```python
from build123d import *

# Parameters (mm, degrees)
SKETCH1_W                = 20
SKETCH1_H                = 70
BOSS_EXTRUDE1_DEPTH      = 10
SKETCH2_W                = 20.25
SKETCH2_H                = 5.1
CUT_EXTRUDE1_DEPTH       = 1
CUT_EXTRUDE1_DEPTH_BACK  = 21
SKETCH3_R                = 4.15
CUT_EXTRUDE2_DEPTH       = 11
BOSS_EXTRUDE2_DEPTH      = 5
BOSS_EXTRUDE2_DEPTH_BACK = 25
CHAMFER1_SIZE            = 1
CHAMFER1_SIZE2           = 0.577350269
CHAMFER1_PART_2_SIZE     = 1
CHAMFER1_PART_2_SIZE2    = 0.577350269


with BuildPart() as part:
    # Sketch1 → Boss-Extrude1 (new body)
    with BuildSketch(Plane(origin=(0, 0, 0), x_dir=(1, 0, 0), z_dir=(0, 1, 0))):
        Rectangle(SKETCH1_W, SKETCH1_H)
    extrude(amount=BOSS_EXTRUDE1_DEPTH)

    # Sketch2 → Cut-Extrude1 (cut, two sides)
    with BuildSketch(Plane(origin=(10, 0, 0), x_dir=(0, 0, -1), z_dir=(1, 0, 0))) as cut_extrude1_sk:
        with Locations((0, 2.55)):
            Rectangle(SKETCH2_W, SKETCH2_H)
    extrude(amount=CUT_EXTRUDE1_DEPTH, mode=Mode.SUBTRACT)
    extrude(cut_extrude1_sk.sketch, amount=-CUT_EXTRUDE1_DEPTH_BACK, mode=Mode.SUBTRACT)

    # Sketch3 → Cut-Extrude2 (cut, through all)
    with BuildSketch(Plane.XZ):
        with Locations((0, 25)):
            Circle(SKETCH3_R)
        with Locations((0, -25)):
            Circle(SKETCH3_R)
    extrude(amount=-CUT_EXTRUDE2_DEPTH, mode=Mode.SUBTRACT)

    # Sketch4 → Boss-Extrude2 (add, two sides)
    with BuildSketch(Plane(origin=(10, 0, 0), x_dir=(0, 0, -1), z_dir=(1, 0, 0))) as boss_extrude2_sk:
        Polygon((-10.125, 0), (-17.525, 0), (-17.525, 10), (17.525, 10), (17.525, 0), (10.125, 0), (10.125, 5.1), (-10.125, 5.1), align=None)
    extrude(amount=BOSS_EXTRUDE2_DEPTH)
    extrude(boss_extrude2_sk.sketch, amount=-BOSS_EXTRUDE2_DEPTH_BACK)

    # Chamfer1
    chamfer1_edges = [part.edges().sort_by_distance(p)[0] for p in [
        (-4.15, 10, 25),
    ]]
    chamfer1_side = [part.faces().sort_by_distance(p)[0] for p in [
        (-4.15, 5, 25),
    ]]
    chamfer(chamfer1_edges, length=CHAMFER1_SIZE, length2=CHAMFER1_SIZE2, reference=chamfer1_side[0])

    # Chamfer1 part 2
    chamfer1_part_2_edges = [part.edges().sort_by_distance(p)[0] for p in [
        (-4.15, 10, -25),
    ]]
    chamfer1_part_2_side = [part.faces().sort_by_distance(p)[0] for p in [
        (-4.15, 5, -25),
    ]]
    chamfer(chamfer1_part_2_edges, length=CHAMFER1_PART_2_SIZE, length2=CHAMFER1_PART_2_SIZE2, reference=chamfer1_part_2_side[0])


solid = part.part
```
Work out the finished part from the listing and answer in its coordinate system (mm). A direction names the side the tool comes from. Round coordinates to 2 decimals unless told otherwise and drop trailing zeros. Order: outer loops, then holes, each group sorted by start corner. A loop starts at its lowest first (then second) coordinate and runs counter-clockwise, first axis right, second up.
Q1. A tool of negligible diameter and unlimited length cuts with its end or side. For faces 1 (the flat face through (12, 5, -17.525)), 2 (the flat face through (-12, 5, -17.525)), 3 (the flat face through (12, 5, 17.525)), 4 (the flat face through (0, 3, 10.125)), 5 (the flat face through (-10, 5, 26)), from which of +Z, -Z, +X, -X, +Y, -Y can it reach the whole face along a straight path? Write none if from no direction.
Solution:
face 1: -Z, +X, +Y, -Y
face 2: -Z, -X, +Y, -Y
face 3: +Z, +X, +Y, -Y
face 4: +X, -X, -Y
face 5: +Z, -X, +Y, -Y
Q2. A cutting plane is placed at C-C, the plane x = 0. Determine the outline of the cut face in (y, z) (3 decimals), then the cut area to 3 significant figures.
Solution:
outline: (0, -35) - (10, -35) - (10, -29.727) - (9, -29.15) - (0, -29.15) - close; (0, -20.85) - (9, -20.85) - (10, -20.273) - (10, 20.273) - (9, 20.85) - (0, 20.85) - (0, 10.125) - (5.1, 10.125) - (5.1, -10.125) - (0, -10.125) - close; (0, 29.15) - (9, 29.15) - (10, 29.727) - (10, 35) - (0, 35) - close
area: 430 mm2
Q3. The mould has two halves that part along X. Classify faces 6 (the flat face through (10, 5, 26)), 7 (the cylindrical face through (-0.9, 4.44, -29.05)), 8 (the flat face through (0, 5, -35)), 9 (the cylindrical face through (-0.9, 4.44, 20.95)): pulls with the +X half, pulls with the -X half, needs draft (parallel to the pull), parting line crosses it, or undercut.
Solution:
face 6: pulls with the +X half
face 7: undercut
face 8: needs draft
face 9: undercut
Q4. Find the intervals of material crossed by line 1 along Z through (x, y) = (0, 4) (3 decimals); line 2 along Z through (x, y) = (0, 5.5); line 3 along Z through (x, y) = (12.75, 3.25) (3 decimals), in increasing order.
Solution:
line 1: z = -35 to -29.15, -20.85 to -10.125, 10.125 to 20.85, 29.15 to 35
line 2: z = -35 to -29.15, -20.85 to 20.85, 29.15 to 35
line 3: z = -17.525 to -10.125, 10.125 to 17.525
Q5. A cutting plane is placed at B-B, the plane z = -25. Determine the outline of the cut face in (x, y).
Solution:
outline: (-10, 0) - (-4.15, 0) - (-4.15, 9) - (-4.73, 10) - (-10, 10) - close; (4.15, 0) - (10, 0) - (10, 10) - (4.73, 10) - (4.15, 9) - close
Q6. A cutting plane is placed at A-A, the plane y = 2.25. Determine the outline of the cut face in (x, z) (3 decimals), then the cut area to 3 significant figures.
Solution:
outline: (-15, -17.525) - (-10, -17.525) - (-10, -35) - (10, -35) - (10, -17.525) - (15, -17.525) - (15, -10.125) - (-15, -10.125) - close; (-15, 10.125) - (15, 10.125) - (15, 17.525) - (10, 17.525) - (10, 35) - (-10, 35) - (-10, 17.525) - (-15, 17.525) - close; hole circle Ø8.3 at (0, -25); hole circle Ø8.3 at (0, 25)
area: 1,030 mm2
Q7. A cutting plane is placed at D-D, the plane y = 8. Determine the outline of the cut face in (x, z) (3 decimals), then the cut area to 3 significant figures.
Solution:
outline: (-15, -17.525) - (-10, -17.525) - (-10, -35) - (10, -35) - (10, -17.525) - (15, -17.525) - (15, 17.525) - (10, 17.525) - (10, 35) - (-10, 35) - (-10, 17.525) - (-15, 17.525) - close; hole circle Ø8.3 at (0, -25); hole circle Ø8.3 at (0, 25)
area: 1,640 mm2
Q8. Given pin 1 Ø5 at (x, z) = (0, 4) entering from -Y; pin 2 Ø3 at (y, z) = (4.5, -29.5) entering from -X; pin 3 Ø1.5 at (x, y) = (11.5, 4) entering from +Z (3 decimals), each flat-ended and moving along its own axis, determine where each tip first touches the part or whether it passes through.
Solution:
pin 1: stops at y = 5.1
pin 2: stops at x = -10
pin 3: stops at z = 17.525
